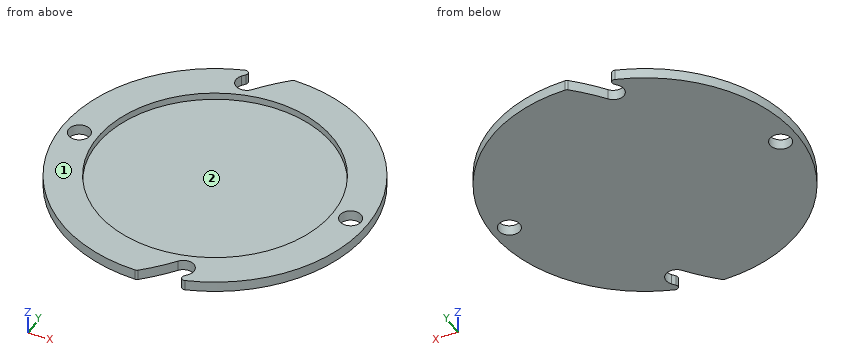
Autodesk Inventor part; units mm, degrees
ref_plane "YZ Plane" through (0, 0, 0) normal (1, 0, 0) x (0, 1, 0)
ref_plane "XZ Plane" through (0, 0, 0) normal (0, 1, 0) x (-1, 0, 0)
ref_plane "XY Plane" through (0, 0, 0) normal (0, 0, 1) x (1, 0, 0)
sketch "スケッチ1" plane through (0, 0, 0) normal (0, 0, 1) x (1, 0, 0)
  circle A0 centre (0, 0) radius 33.5 construction
  circle A1 centre (0, 0) radius 43.5
  dimension "d0" = 67
  dimension "d1" = 87
extrude "押し出し1" add sketch "スケッチ1" along normal blind 1
sketch "スケッチ2" plane through (0, 0, 1) normal (0, 0, 1) x (1, 0, 0)
  circle A0 centre (0, 0) radius 33.5
  circle A1 centre (0, 0) radius 43.5
  dimension "d4" = 67
extrude "押し出し2" add sketch "スケッチ2" along normal blind 2
sketch "スケッチ4" plane through (0, 0, 3) normal (0, 0, 1) x (1, 0, 0)
  circle A0 centre (0, 0) radius 33.5 construction
  circle A1 centre (0, 0) radius 43.5 construction
  line L0 (0, 0) -> (33.5, 0) construction
  line L1 (33.5, 0) -> (43.5, 0) construction
  circle A2 centre (0, 0) radius 33.5 construction
  line L2 (0, 0) -> (-33.5, 0) construction
  circle A3 centre (0, 0) radius 43.5 construction
  line L3 (-43.5, 0) -> (-33.5, 0) construction
  circle A4 centre (38.5, 0) radius 3.05
  circle A5 centre (-38.5, 0) radius 3.05
  circle A6 centre (0, 0) radius 38.5 construction
  circle A7 centre (-9.9645, 37.1881) radius 3.05 construction
  arc A8 (-3.4944, 44.3648) -> (-9.9645, 37.1881) centre (38.5, 0) ccw construction
  line L4 (38.5, 0) -> (-9.9645, 37.1881) construction
  line L5 (-9.9645, 37.1881) -> (-12.3843, 39.0449) construction
  arc A9 (0.0788, 43.4999) -> (-7.5448, 35.3314) centre (38.5, 0) ccw
  arc A10 (-9.6001, 42.4274) -> (-12.3843, 39.0449) centre (38.5, 0) ccw
  arc A11 (-12.3843, 39.0449) -> (-7.5448, 35.3314) centre (-9.9645, 37.1881) ccw
  arc A12 (0.0788, 43.4999) -> (-9.6001, 42.4274) centre (0, 0) ccw
  circle A13 centre (9.9645, -37.1881) radius 3.05 construction
  line L6 (-38.5, 0) -> (9.9645, -37.1881) construction
  line L7 (9.9645, -37.1881) -> (12.3843, -39.0449) construction
  arc A14 (-0.0788, -43.4999) -> (7.5448, -35.3314) centre (-38.5, 0) ccw
  arc A15 (9.6001, -42.4274) -> (12.3843, -39.0449) centre (-38.5, 0) ccw
  arc A16 (12.3843, -39.0449) -> (7.5448, -35.3314) centre (9.9645, -37.1881) ccw
  arc A17 (-0.0788, -43.4999) -> (9.6001, -42.4274) centre (0, 0) ccw
  line L8 (-9.9645, 37.1881) -> (9.9645, -37.1881) construction
  dimension "d7" = 6.1
  dimension "d8" = 3.05
  dimension "d15" = 105
extrude "押し出し3" cut sketch "スケッチ4" against normal through all
fillet "フィレット1" radius 1 4 edges at (-9.6001, 42.4274, 1.5) (0.0788, 43.4999, 1.5) (-0.0788, -43.4999, 1.5) (9.6001, -42.4274, 1.5)
properties part number "kanure_01"
CAD build for the part. Positions are in the model's coordinates, mm. Face numbers are marked on the shaded views. Round coordinates to 2 decimals unless told otherwise and drop trailing zeros. Loops run counter-clockwise (first coordinate to the right, second up) from the corner with the lowest first, then second, coordinate; pieces in that order, holes last.
(1) Cut at A-A (x = -38.5). Give the cut face in (y, z).
(2) Two-plate mould, pull along Y, no slides. Class the marked faces 1 and 2: +Y half, -Y half, draft (parallel to the pull), parting line (faces both ways), or undercut.
(3) Cut at B-B (y = 21). Give the cut face in (x, z), plus the area to 3 significant figures.
(4) Cut at C-C (z = 2.1). State how many separate pieces and enclosed holes the cut face has, plus the area to 3 significant figures.
(5) Drop flat-ended pins along their axis: pin 1 (1.5 mm diameter, centred on y = -26, z = 1.5, fed in from +X); pin 2 (1.5 mm diameter, centred on x = 30.5, z = 2.5, fed in from +Y). Give the stop position or say it passes through.
(6) Cut at D-D (x = 31.5). Give the cut face in (y, z), plus the area to 3 significant figures.
(7) Wall check: line 1 along Z through (x, y) = (6.5, 3); line 2 along X through (y, z) = (4, 2.1); line 3 along Y through (x, z) = (38, 0.6). Give the ranges that are in metal, low to high.
Findings below:
1. outline: (-20.25, 0) - (-3.05, 0) - (-3.05, 3) - (-20.25, 3) - close; (3.05, 0) - (20.25, 0) - (20.25, 3) - (3.05, 3) - close
2. face 1: draft
2. face 2: undercut
3. outline: (-38.1, 0) - (38.1, 0) - (38.1, 3) - (26.1, 3) - (26.1, 1) - (-26.1, 1) - (-26.1, 3) - (-38.1, 3) - close
3. area: 124 mm2
4. separate pieces: 1
4. enclosed holes: 3
4. area: 2,230 mm2
5. pin 1: stops at x = 35.42
5. pin 2: stops at y = 31.74
6. outline: (-30, 0) - (30, 0) - (30, 3) - (11.4, 3) - (11.4, 1) - (-11.4, 1) - (-11.4, 3) - (-30, 3) - close
6. area: 134 mm2
7. line 1: z = 0 to 1
7. line 2: x = -43.32 to -33.26, 33.26 to 43.32
7. line 3: y = -21.17 to -3.01, 3.01 to 21.17
